Build history of the part. All positions in model axes, mm. A direction names the side the tool comes from. Round coordinates to 2 decimals unless told otherwise and drop trailing zeros. Write each loop counter-clockwise with the first axis right and the second up, starting at its lowest first coordinate (ties: lowest second). Pieces come first, ordered by that corner, then holes. Notation, with made-up numbers: (-33, 15.5) -> (-25, 15.5) arc R30 ccw to (-25, 46.5) -> close; hole circle Ø8 at (-19.5, 33.5). An arc over 180 degrees is marked (long way). Answer as CSV lines item,"result".
from build123d import *

# Parameters (mm, degrees)
SKETCH_1_W                    = 480
SKETCH_1_H                    = 94
EXTRUDE_1_DEPTH               = 40
SKETCH_2_W                    = 40
SKETCH_2_H                    = 20
CUT_EXTRUDE_1_DEPTH           = 259.526594377
SKETCH_3_W                    = 360
SKETCH_3_H                    = 20
CUT_EXTRUDE_2_DEPTH           = 259.526594377
SKETCH_4_W                    = 40
SKETCH_4_H                    = 20
CUT_EXTRUDE_3_DEPTH           = 259.526594377
HOLE_WIZARD_M10_1_D           = 11
HOLE_WIZARD_M10_1_CBORE_D     = 18
HOLE_WIZARD_M10_1_CBORE_DEPTH = 11
SKETCH_14_W                   = 373.229690018
SKETCH_14_H                   = 73.09887193
EXTRUDE_2_DEPTH               = 74.29
SKETCH_15_W                   = 278.085126552
SKETCH_15_H                   = 48.34581477
CUT_EXTRUDE_4_DEPTH           = 74.29


with BuildPart() as part:
    # 草图1 → 凸台-拉伸1 (new body)
    with BuildSketch(Plane.XZ.offset(20)):
        Rectangle(SKETCH_1_W, SKETCH_1_H)
    extrude(amount=-EXTRUDE_1_DEPTH)

    # 草图2 → 切除-拉伸1 (cut, through all)
    with BuildSketch(Plane(origin=(0, 0, -47), x_dir=(-1, 0, 0), z_dir=(0, 0, -1))):
        with Locations((220, 10)):
            Rectangle(SKETCH_2_W, SKETCH_2_H)
    extrude(amount=-CUT_EXTRUDE_1_DEPTH, mode=Mode.SUBTRACT)

    # 草图3 → 切除-拉伸2 (cut, through all)
    with BuildSketch(Plane(origin=(0, 0, -47), x_dir=(-1, 0, 0), z_dir=(0, 0, -1))):
        with Locations((0, -10)):
            Rectangle(SKETCH_3_W, SKETCH_3_H)
    extrude(amount=-CUT_EXTRUDE_2_DEPTH, mode=Mode.SUBTRACT)

    # 草图4 → 切除-拉伸3 (cut, through all)
    with BuildSketch(Plane(origin=(0, 0, -47), x_dir=(-1, 0, 0), z_dir=(0, 0, -1))):
        with Locations((-220, 10)):
            Rectangle(SKETCH_4_W, SKETCH_4_H)
    extrude(amount=-CUT_EXTRUDE_3_DEPTH, mode=Mode.SUBTRACT)

    # M10 六角头螺栓的柱形沉头孔1 (through all)
    with Locations(Plane(origin=(0, 0, 0), x_dir=(1, 0, 0), z_dir=(0, 1, 0))):
        with Locations((220, -27), (220, 27), (-220, -27), (-220, 27)):
            CounterBoreHole(HOLE_WIZARD_M10_1_D / 2, HOLE_WIZARD_M10_1_CBORE_D / 2, HOLE_WIZARD_M10_1_CBORE_DEPTH)

    # 草图14 → 凸台-拉伸2 (add)
    with BuildSketch(Plane(origin=(0, 20, 0), x_dir=(1, 0, 0), z_dir=(0, 1, 0))):
        Rectangle(SKETCH_14_W, SKETCH_14_H)
    extrude(amount=EXTRUDE_2_DEPTH)

    # 草图15 → 切除-拉伸4 (cut)
    with BuildSketch(Plane(origin=(0, 94.29, 0), x_dir=(1, 0, 0), z_dir=(0, 1, 0))):
        Rectangle(SKETCH_15_W, SKETCH_15_H)
    extrude(amount=-CUT_EXTRUDE_4_DEPTH, mode=Mode.SUBTRACT)


solid = part.part
1. Cut at A-A, the plane x = 220. Write the cut outline in (y, z).
Results found:
outline,"(-20, -47) -> (0, -47) -> (0, -36) -> (-11, -36) -> (-11, -32.5) -> (-20, -32.5) -> close; (-20, -21.5) -> (-11, -21.5) -> (-11, -18) -> (0, -18) -> (0, 18) -> (-11, 18) -> (-11, 21.5) -> (-20, 21.5) -> close; (-20, 32.5) -> (-11, 32.5) -> (-11, 36) -> (0, 36) -> (0, 47) -> (-20, 47) -> close"
2. Which spindle directions (+Z, -Z, +X, -X, +Y, -Y) get a long thin tool onto all of the face, cutting with end or side? Do faces 1 (the flat face through (-224, -11, 31)), 2 (the flat face through (-3, 57, 36.549)), 3 (the flat face through (-200, 10, -1)), 4 (the flat face through (-210, -20, 1)), 5 (the flat face through (-3, 57, -36.549)). Say none if no direction does.
Results found:
face 1,"+Y"
face 2,"+Z, +X, -X, +Y"
face 3,"+Z, -Z, -X, +Y"
face 4,"+Z, -Z, +X, -X, -Y"
face 5,"-Z, +X, -X, +Y"
3. Cut at D-D, the plane z = 8.5. Write the cut outline in (x, y).
Results found:
outline,"(-240, -20) -> (-180, -20) -> (-180, 0) -> (180, 0) -> (180, -20) -> (240, -20) -> (240, 0) -> (200, 0) -> (200, 20) -> (186.61, 20) -> (186.61, 94.29) -> (139.04, 94.29) -> (139.04, 20) -> (-139.04, 20) -> (-139.04, 94.29) -> (-186.61, 94.29) -> (-186.61, 20) -> (-200, 20) -> (-200, 0) -> (-240, 0) -> close"
4. Mould opens along Z. For faces 6 (the cylindrical face through (211, -5, -27)), 7 (the flat face through (200, 10, -1)), 8 (the flat face through (-3, 4, 47)), 9 (the cylindrical face through (-214.505, -15.563, -27.242)) say: +Z half, -Z half, draft (parallel to the pull), parting line (faces both ways), or undercut.
Results found:
face 6,"undercut"
face 7,"draft"
face 8,"+Z half"
face 9,"undercut"
5. Cut at B-B, the plane y = 57. Write the cut outline in (x, z).
Results found:
outline,"(-186.61, -36.55) -> (186.61, -36.55) -> (186.61, 36.55) -> (-186.61, 36.55) -> close; hole (-139.04, -24.17) -> (139.04, -24.17) -> (139.04, 24.17) -> (-139.04, 24.17) -> close"
6. Cut at C-C, the plane x = -86.5. Write the cut outline in (y, z).
Results found:
outline,"(0, -47) -> (20, -47) -> (20, -36.55) -> (94.29, -36.55) -> (94.29, -24.17) -> (20, -24.17) -> (20, 24.17) -> (94.29, 24.17) -> (94.29, 36.55) -> (20, 36.55) -> (20, 47) -> (0, 47) -> close"
7. Probe line 1 along Z through (x, y) = (-220, -17); line 2 along X through (y, z) = (-17.25, -27); line 3 along Z through (x, y) = (-220, -5.75). List the from-to ranges inside material, lowest first.
Results found:
line 1,"z = -47 to -32.5, -21.5 to 21.5, 32.5 to 47"
line 2,"x = -240 to -225.5, -214.5 to -180, 180 to 214.5, 225.5 to 240"
line 3,"z = -47 to -36, -18 to 18, 36 to 47"
8. Drop flat-ended pins along their axis: pin 1 Ø22.5 at (x, y) = (26, 64.5) entering from -Z; pin 2 Ø3 at (x, y) = (-37, 71) entering from +Z; pin 3 Ø14.5 at (x, z) = (21, 6.5) entering from +Y; pin 4 Ø10 at (x, z) = (220, -27) entering from +Y. Give the stop position or say it passes through.
Results found:
pin 1,"stops at z = -36.55"
pin 2,"stops at z = 36.55"
pin 3,"stops at y = 20"
pin 4,"passes through"
